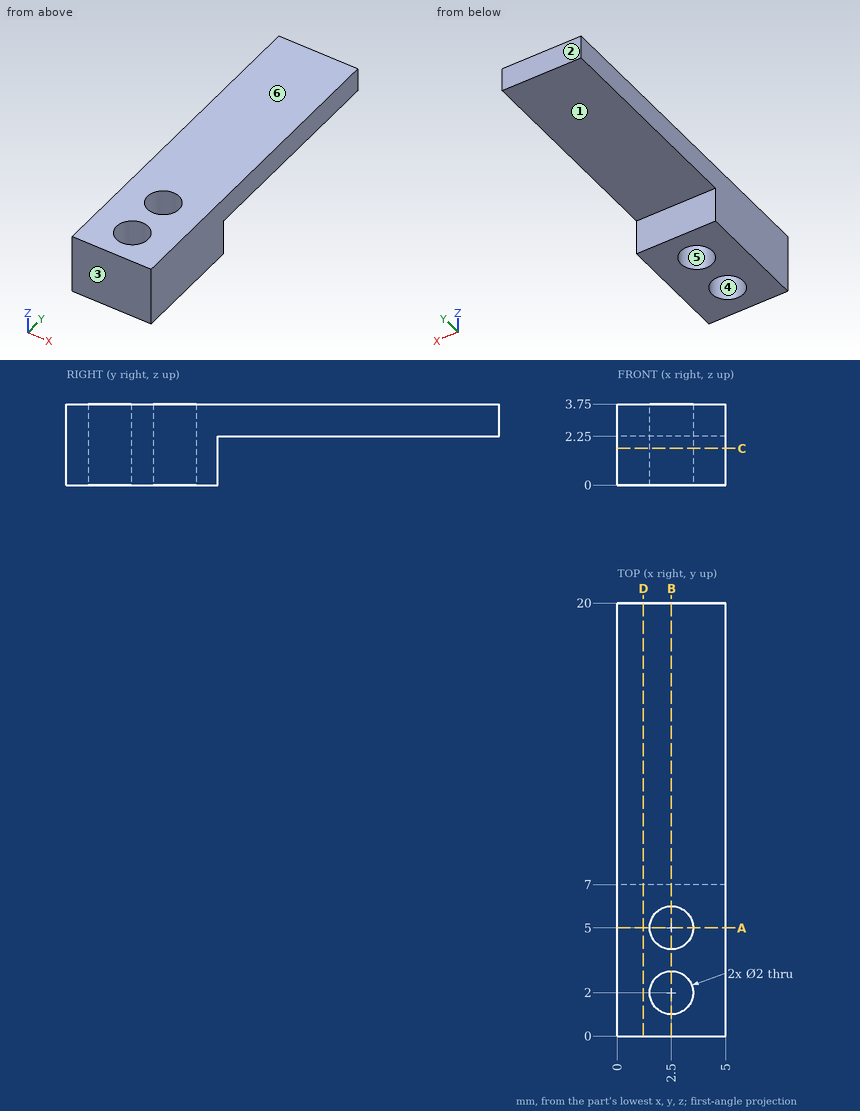
Source: three-view drawing plus pictorial views. Frame: mm from the lowest corner of the part. A direction names the side the tool comes from. Coordinates: 2 decimals unless noted, no trailing zeros. Order: outer loops, then holes, each group sorted by start corner. A loop starts at its lowest first (then second) coordinate and runs counter-clockwise, first axis right, second up. Notation, with made-up numbers: M 84.25,1.5 L 98.25,1.5 A11 ccw 98.25,15.5 Z; hole C 8.25,46.25 d5. An arc over 180 degrees is marked long. One line per question, with ' | ' between items. Start each with the question number.
Item 1: Set-up query: the marked faces 1 and 2. Return all of +Z, -Z, +X, -X, +Y, -Y with unobstructed straight access to the full face (end or side cutting, diameter ignored); none if empty.
Item 2: Pin query (flat end, axial travel): pin 1 Ø0.7 at (x, z) = (2.5, 1.5) entering from +Y. Return the tip coordinate at first contact, or that it passes through.
Item 3: Draft query along Y for the marked faces 3, 4, 5 and 6. Return one class per face: released by +Y, released by -Y, zero draft, split by the parting line, or undercut.
Item 4: Ray query, probe 1 along Y at (x, z) = (2.5, 1.95); probe 2 along Z at (x, y) = (1.8, 17.5); probe 3 along Y at (x, z) = (1.8, 1.65). Return the intervals inside material, ascending. Write a range as [from, to].
Item 5: Cut plane C-C, the plane z = 1.7. Return the cut outline in (x, y), then the cut area to 3 significant figures.
Item 6: Cut plane A-A, the plane y = 5. Return the cut outline in (x, z), then the cut area to 4 significant figures.
Item 7: Cut plane D-D, the plane x = 1.2. Return the cut outline in (y, z), then the cut area to 4 significant figures.
Item 8: Cut plane B-B, the plane x = 2.5. Return the cut outline in (y, z).
A:
1) face 1: -Z, +X, -X, +Y | face 2: +Z, -Z, +X, -X, +Y
2) pin 1: stops at y = 7
3) face 3: released by -Y | face 4: undercut | face 5: undercut | face 6: zero draft
4) probe 1: y = [0, 1], [3, 4], [6, 7] | probe 2: z = [2.25, 3.75] | probe 3: y = [0, 1.29], [2.71, 4.29], [5.71, 7]
5) outline: M 0,0 L 5,0 L 5,7 L 0,7 Z; hole C 2.5,2 d2; hole C 2.5,5 d2 | area: 28.7 mm2
6) outline: M 0,0 L 1.5,0 L 1.5,3.75 L 0,3.75 Z; M 3.5,0 L 5,0 L 5,3.75 L 3.5,3.75 Z | area: 11.25 mm2
7) outline: M 0,0 L 7,0 L 7,2.25 L 20,2.25 L 20,3.75 L 0,3.75 Z | area: 45.75 mm2
8) outline: M 0,0 L 1,0 L 1,3.75 L 0,3.75 Z; M 3,0 L 4,0 L 4,3.75 L 3,3.75 Z; M 6,0 L 7,0 L 7,2.25 L 20,2.25 L 20,3.75 L 6,3.75 Z
